```python
from build123d import *

# Parameters (mm, degrees)
BOSS_EXTRUDE1_DEPTH             = 90
BOSS_EXTRU_2_DEPTH              = 180
BOSS_EXTRUDE2_DEPTH             = 180
DIAM_TRE_DU_PER_AGE_4_5_4_5_1_D = 4.5
DIAM_TRE_DU_PER_AGE_4_0_4_1_D   = 4
F_4_5_4_5_DIAMETER_HOLE1_D      = 4.5
BOSS_EXTRU_1_DEPTH              = 30
BOSS_EXTRU_3_DEPTH              = 30
SYM_TRIE2_START                 = 6.1
SYM_TRIE2_OUTLINE_R             = 2.25
SYM_TRIE2_DEPTH                 = 13.898019485
DIAM_TRE_DU_PER_AGE_4_5_4_5_4_D = 4.5
ESQUISSE15_W                    = 5.4
ESQUISSE15_H                    = 1.96
BOSS_EXTRU_4_DEPTH              = 180


# Read off the part's stored shape, not the designer's step: Symétrie2
with BuildPart() as part:
    # Sketch5 → Boss-Extrude1 (new, symmetric)
    with BuildSketch(Plane(origin=(0, 0, 0), x_dir=(0, 0, -1), z_dir=(1, 0, 0))):
        with BuildLine():
            Line((-19.998019485, 4.9), (-18.198019485, 3.1))
            Line((-18.198019485, 3.1), (-18.198019485, 5.499339828))
            Line((-18.198019485, 5.499339828), (-16.558019485, 5.499339828))
            Line((-16.558019485, 5.499339828), (-13.9, 2.841320344))
            Line((-13.9, 2.841320344), (-13.9, -2.838679656))
            Line((-13.9, -2.838679656), (-16.558019485, -5.496699141))
            Line((-16.558019485, -5.496699141), (-18.198019485, -5.496699141))
            Line((-18.198019485, -5.496699141), (-18.198019485, -3.1))
            Line((-18.198019485, -3.1), (-19.998019485, -4.9))
            Line((-19.998019485, -4.9), (-19.998019485, -9))
            ThreePointArc((-19.998019485, -9), (-19.705126266, -9.707106781), (-18.998019485, -10))
            Line((-18.998019485, -10), (-14.9, -10))
            Line((-14.9, -10), (-13.1, -8.2))
            Line((-13.1, -8.2), (-15.5, -8.2))
            Line((-15.5, -8.2), (-15.5, -6.56))
            Line((-15.5, -6.56), (-12.84, -3.9))
            Line((-12.84, -3.9), (-7.16, -3.9))
            Line((-7.16, -3.9), (-4.5, -6.56))
            Line((-4.5, -6.56), (-4.5, -8.2))
            Line((-4.5, -8.2), (-6.9, -8.2))
            Line((-6.9, -8.2), (-5.1, -10))
            Line((-5.1, -10), (5.1, -10))
            Line((5.1, -10), (6.9, -8.2))
            Line((6.9, -8.2), (4.496038969, -8.2))
            Line((4.496038969, -8.2), (4.496038969, -6.56))
            Line((4.496038969, -6.56), (7.156038969, -3.9))
            Line((7.156038969, -3.9), (12.836038969, -3.9))
            Line((12.836038969, -3.9), (15.496038969, -6.56))
            Line((15.496038969, -6.56), (15.496038969, -8.2))
            Line((15.496038969, -8.2), (13.1, -8.2))
            Line((13.1, -8.2), (14.9, -10))
            Line((14.9, -10), (19.001980515, -10))
            ThreePointArc((19.001980515, -10), (19.709087297, -9.707106781), (20.001980515, -9))
            Line((20.001980515, -9), (20.001980515, -4.9))
            Line((20.001980515, -4.9), (18.201980515, -3.1))
            Line((18.201980515, -3.1), (18.201980515, -5.504621202))
            Line((18.201980515, -5.504621202), (16.561980515, -5.504621202))
            Line((16.561980515, -5.504621202), (13.9, -2.842640687))
            Line((13.9, -2.842640687), (13.9, 2.837359313))
            Line((13.9, 2.837359313), (16.561980515, 5.499339828))
            Line((16.561980515, 5.499339828), (18.201980515, 5.499339828))
            Line((18.201980515, 5.499339828), (18.201980515, 3.1))
            Line((18.201980515, 3.1), (20.001980515, 4.9))
            Line((20.001980515, 4.9), (20.001980515, 9))
            ThreePointArc((20.001980515, 9), (19.709087297, 9.707106781), (19.001980515, 10))
            Line((19.001980515, 10), (14.9, 10))
            Line((14.9, 10), (13.1, 8.2))
            Line((13.1, 8.2), (15.501320344, 8.2))
            Line((15.501320344, 8.2), (15.501320344, 6.56))
            Line((15.501320344, 6.56), (12.841320344, 3.9))
            Line((12.841320344, 3.9), (7.161320344, 3.9))
            Line((7.161320344, 3.9), (4.501320344, 6.56))
            Line((4.501320344, 6.56), (4.501320344, 8.2))
            Line((4.501320344, 8.2), (6.9, 8.2))
            Line((6.9, 8.2), (5.1, 10))
            Line((5.1, 10), (-5.1, 10))
            Line((-5.1, 10), (-6.9, 8.2))
            Line((-6.9, 8.2), (-4.501320344, 8.2))
            Line((-4.501320344, 8.2), (-4.501320344, 6.56))
            Line((-4.501320344, 6.56), (-7.161320344, 3.9))
            Line((-7.161320344, 3.9), (-12.841320344, 3.9))
            Line((-12.841320344, 3.9), (-15.501320344, 6.56))
            Line((-15.501320344, 6.56), (-15.501320344, 8.2))
            Line((-15.501320344, 8.2), (-13.1, 8.2))
            Line((-13.1, 8.2), (-14.9, 10))
            Line((-14.9, 10), (-18.998019485, 10))
            ThreePointArc((-18.998019485, 10), (-19.705126266, 9.707106781), (-19.998019485, 9))
            Line((-19.998019485, 9), (-19.998019485, 4.9))
        make_face()
        Polygon((6.1, -2.84), (6.1, 2.84), (2.7, 6.24), (2.7, 8.2), (-2.7, 8.2), (-2.7, 6.24), (-6.1, 2.84), (-6.1, -2.84), (-2.7, -6.24), (-2.7, -8.2), (2.7, -8.2), (2.7, -6.24), align=None, mode=Mode.SUBTRACT)
    extrude(amount=BOSS_EXTRUDE1_DEPTH, both=True)

    # Esquisse10 → Boss.-Extru.2 (add, through all)
    with BuildSketch(Plane(origin=(90, 0, 0), x_dir=(0, 0, -1), z_dir=(1, 0, 0))):
        Polygon((-19.998019485, 4.9), (-19.998019485, -4.9), (-18.198019485, -3.1), (-18.198019485, -5.496699141), (-16.558019485, -5.496699141), (-13.9, -2.838679656), (-13.9, 2.841320344), (-16.558019485, 5.499339828), (-18.198019485, 5.499339828), (-18.198019485, 3.1), align=None)
    extrude(amount=-BOSS_EXTRU_2_DEPTH)

    # Sketch6 → Boss-Extrude2 (add)
    with BuildSketch(Plane.ZY.offset(90)):
        Polygon((5.1, 10), (14.9, 10), (13.1, 8.2), (15.501320344, 8.2), (15.501320344, 6.56), (12.841320344, 3.9), (7.161320344, 3.9), (4.501320344, 6.56), (4.501320344, 8.2), (6.9, 8.2), align=None)
    boss_extrude2 = extrude(amount=-BOSS_EXTRUDE2_DEPTH)

    # Diamètre du perçage Ø4.5 (4.5)1 (through all)
    with Locations(Plane(origin=(0, 0, -13.9), x_dir=(-1, 0, 0), z_dir=(0, 0, -1))):
        with Locations((85, -0.002640687), (73, -0.002640687), (61, -0.002640687), (49, -0.002640687)):
            Hole(DIAM_TRE_DU_PER_AGE_4_5_4_5_1_D / 2)

    # Diamètre du perçage Ø4.0 (4)1 (through all)
    with Locations(Plane(origin=(0, -3.9, 0), x_dir=(-1, 0, 0), z_dir=(0, -1, 0))):
        with Locations((44, 9.996038969), (80, 9.996038969), (68, 9.996038969), (56, 9.996038969)):
            Hole(DIAM_TRE_DU_PER_AGE_4_0_4_1_D / 2)

    # Mirror1: Boss-Extrude2 across plane
    add(boss_extrude2.mirror(Plane.ZX))

    # Ø4.5 (4.5) Diameter Hole1 (through all)
    with Locations(Plane(origin=(0, 10, 0), x_dir=(-1, 0, 0), z_dir=(0, 1, 0))):
        with Locations((80, 7.160660172), (44, 7.160660172), (56, 7.160660172), (68, 7.160660172)):
            Hole(F_4_5_4_5_DIAMETER_HOLE1_D / 2)

    # Esquisse7 → Boss.-Extru.1 (add)
    with BuildSketch(Plane(origin=(90, 0, 0), x_dir=(0, 0, -1), z_dir=(1, 0, 0))):
        Polygon((14.9, -10), (5.1, -10), (6.9, -8.2), (4.496038969, -8.2), (4.496038969, -6.56), (7.156038969, -3.9), (12.836038969, -3.9), (15.496038969, -6.56), (15.496038969, -8.2), (13.1, -8.2), align=None)
    extrude(amount=-BOSS_EXTRU_1_DEPTH)

    # Esquisse11 → Boss.-Extru.3 (add)
    with BuildSketch(Plane(origin=(90, 0, 0), x_dir=(0, 0, -1), z_dir=(1, 0, 0))):
        Polygon((14.9, 10), (5.1, 10), (6.9, 8.2), (4.501320344, 8.2), (4.501320344, 6.56), (7.161320344, 3.9), (12.841320344, 3.9), (15.501320344, 6.56), (15.501320344, 8.2), (13.1, 8.2), align=None)
    extrude(amount=-BOSS_EXTRU_3_DEPTH)

    # Symétrie2 outline → Symétrie2 (cut)
    with BuildSketch(Plane.XY.offset(SYM_TRIE2_START)):
        with Locations((49, -0.002640687)):
            Circle(SYM_TRIE2_OUTLINE_R)
        with Locations((61, -0.002640687)):
            Circle(SYM_TRIE2_OUTLINE_R)
        with Locations((73, -0.002640687)):
            Circle(SYM_TRIE2_OUTLINE_R)
        with Locations((85, -0.002640687)):
            Circle(SYM_TRIE2_OUTLINE_R)
    extrude(amount=SYM_TRIE2_DEPTH, mode=Mode.SUBTRACT)

    # Diamètre du perçage Ø4.5 (4.5)4 (through all)
    with Locations(Plane(origin=(0, 10, 0), x_dir=(1, 0, 0), z_dir=(0, 1, 0))):
        with Locations((65, 10.001320344), (85, 10.001320344)):
            Hole(DIAM_TRE_DU_PER_AGE_4_5_4_5_4_D / 2)

    # Esquisse15 → Boss.-Extru.4 (add, through all)
    with BuildSketch(Plane.ZY.offset(90)):
        with Locations((0, -7.22)):
            Rectangle(ESQUISSE15_W, ESQUISSE15_H)
        with Locations((0, 7.22)):
            Rectangle(ESQUISSE15_W, ESQUISSE15_H)
        Polygon((-18.201980515, -3.1), (-16.561980515, -5.504621202), (-18.201980515, -5.504621202), align=None)
        Polygon((-18.201980515, 3.1), (-16.561980515, 5.499339828), (-18.201980515, 5.499339828), align=None)
    extrude(amount=-BOSS_EXTRU_4_DEPTH)


solid = part.part
```
Input: part model. Units: mm. Frame: model coordinates. A direction names the side the tool comes from. Give positions to 0.01 mm unless a question says otherwise; leave off trailing zeros. Answer as CSV lines item,"result". Start each with the question number.
1. Reachability of faces 5 (the face through (-63.248, 0.096, 13.146)), 6 (the face through (75.08, -0.86, 12.95)), 7 (the face through (1, 0, -6.1)) from +Z, -Z, +X, -X, +Y, -Y: full face, straight path, thin tool, end or side. Return the list, or none.
2. Line query: L1, parallel to Z at x = -56, y = -1.5; L2, parallel to Z at x = -17, y = 5.75; L3, parallel to X at y = 8, z = -8. Output: solid intervals per line, ascending.
3. Section A-A on x = 65. State how many separate pieces and enclosed holes the cut face has, plus the area to 3 significant figures.
4. Pull-direction query (Y, two-part tool) for faces 1 (the face through (-76, 0, 6.1)), 2 (the face through (-14, 3.9, -10)), 3 (the face through (-90, 0, 9)), 4 (the face through (-70.92, -0.86, 13.15)); classes: released by +Y, released by -Y, zero draft, split by the parting line, or undercut.
5. Pin query (flat end, axial travel): P1, Ø5, axis at x = 49, y = 0, coming from the -Z side; P2, Ø3, axis at x = -44, z = -10, coming from the -Y side; P3, Ø5, axis at x = -61, y = 0, coming from the +Z side; P4, Ø6, axis at x = -62.5, y = 1, coming from the -Z side. Return the tip coordinate at first contact, or that it passes through.
Computed values:
1,face 5,"+Z, -Z"
1,face 6,"+Z"
1,face 7,"+X, -X"
2,L1,"z = -13.9 to -12, -8 to -6.1, 9.41 to 20"
2,L2,"z = -20 to -14.69, -5.31 to -3.19, 3.19 to 20"
2,L3,"x = 60 to 63.97, 66.03 to 83.97, 86.03 to 90"
3,separate pieces,"2"
3,enclosed holes,"2"
3,area,"529 mm²"
4,face 1,"undercut"
4,face 2,"released by +Y"
4,face 3,"zero draft"
4,face 4,"undercut"
5,P1,"stops at z = -13.9"
5,P2,"passes through"
5,P3,"stops at z = 20"
5,P4,"stops at z = -19.1"
